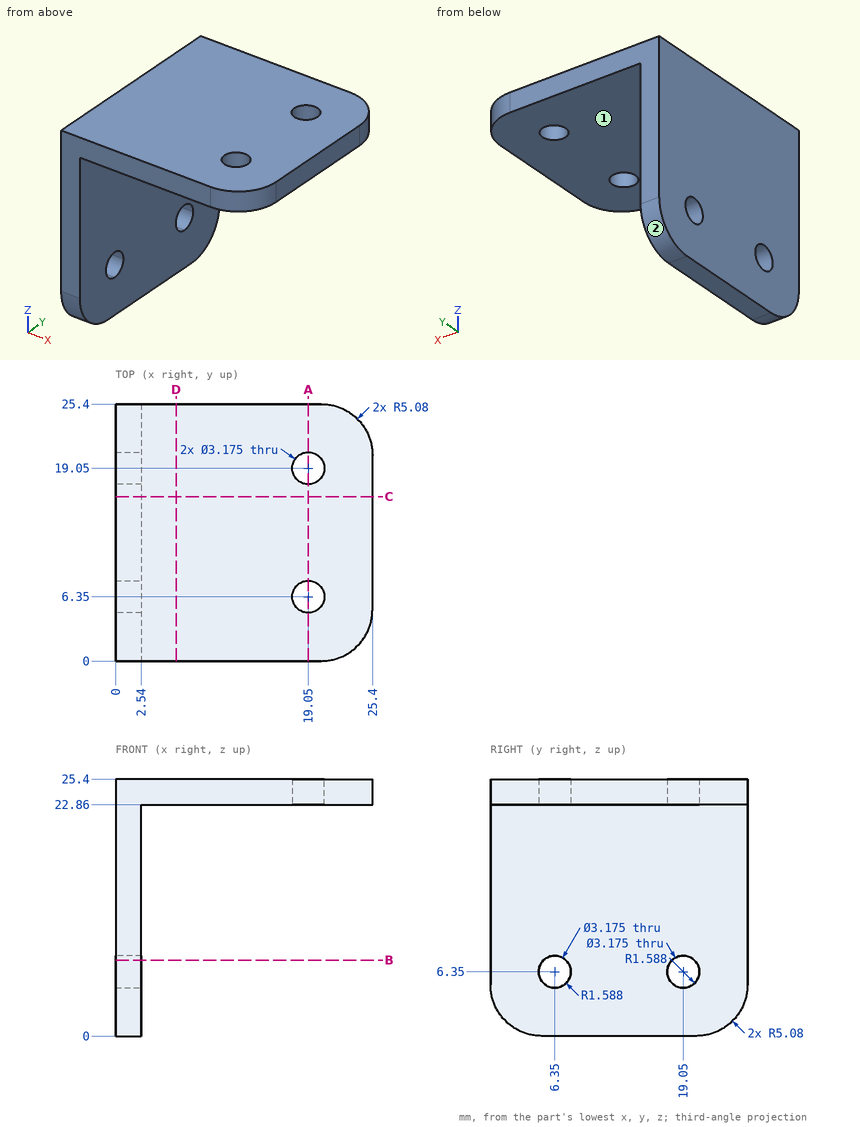
Input: dimensioned drawing with shaded views. Units: mm. Origin: part minimum x, y, z. A direction names the side the tool comes from. Give positions to 0.01 mm unless a question says otherwise; leave off trailing zeros. Loops run counter-clockwise (first coordinate to the right, second up) from the corner with the lowest first, then second, coordinate; pieces in that order, holes last. Notation, with made-up numbers: (52.5, -37) -> (67.5, -37) arc R26 cw to (67.5, -11) -> close; hole circle Ø2 at (27, -33). An arc over 180 degrees is marked (long way). Return JSON: item names as keys, results as strings.
Item 1: Section B-B, the plane z = 7.5. Output: boundary loops of the cut face in (x, y) (1 decimal).
Filled in:
{"outline": "(0, 0) -> (2.5, 0) -> (2.5, 5.3) -> (0, 5.3) -> close; (0, 7.4) -> (2.5, 7.4) -> (2.5, 18) -> (0, 18) -> close; (0, 20.1) -> (2.5, 20.1) -> (2.5, 25.4) -> (0, 25.4) -> close"}
Item 2: Access query for the marked faces 1 and 2. Directions: +Z, -Z, +X, -X, +Y, -Y. A direction counts if a zero-diameter tool reaches every point of the face in a straight line with its end or side. Return the directions, or none.
Filled in:
{"face 1": "-Z, +X, +Y, -Y", "face 2": "-Z, +X, -X, +Y"}
Item 3: Line query: line 1 (Y direction, x = 19.05, z = 23.65); line 2 (Z direction, x = 1.3, y = 6.35); line 3 (X direction, y = 19.05, z = 24.7). Output: solid intervals per line, ascending.
Filled in:
{"line 1": "0 to 4.76, 7.94 to 17.46, 20.64 to 25.4", "line 2": "0 to 4.76, 7.94 to 25.4", "line 3": "0 to 17.46, 20.64 to 25.4"}
Item 4: Pin query (flat end, axial travel): P1, Ø8, axis at x = 18, y = 3, coming from the -Z side; P2, Ø1, axis at y = 19, z = 4.5, coming from the +X side. Return the tip coordinate at first contact, or that it passes through.
Filled in:
{"P1": "z = 22.86", "P2": "x = 2.54"}
Item 5: Section D-D, the plane x = 6. Output: boundary loops of the cut face in (y, z).
Filled in:
{"outline": "(0, 22.86) -> (25.4, 22.86) -> (25.4, 25.4) -> (0, 25.4) -> close"}
Item 6: Section A-A, the plane x = 19.05. Output: boundary loops of the cut face in (y, z).
Filled in:
{"outline": "(0, 22.86) -> (4.76, 22.86) -> (4.76, 25.4) -> (0, 25.4) -> close; (7.94, 22.86) -> (17.46, 22.86) -> (17.46, 25.4) -> (7.94, 25.4) -> close; (20.64, 22.86) -> (25.4, 22.86) -> (25.4, 25.4) -> (20.64, 25.4) -> close"}
Item 7: Section C-C, the plane y = 16.25. Output: boundary loops of the cut face in (x, z).
Filled in:
{"outline": "(0, 0) -> (2.54, 0) -> (2.54, 22.86) -> (25.4, 22.86) -> (25.4, 25.4) -> (0, 25.4) -> close"}
